The listing builds one solid part. Answer for the finished solid, in the listing's coordinates (mm). Coordinates: 2 decimals unless noted, no trailing zeros. Order: outer loops, then holes, each group sorted by start corner. A loop starts at its lowest first (then second) coordinate and runs counter-clockwise, first axis right, second up. Notation, with made-up numbers: (73.5, 57.25) -> (82.5, 57.25) arc R32 cw to (82.5, 90.25) -> close; hole circle Ø9 at (38, 51). An arc over 180 degrees is marked (long way). One line per question, with ' | ' between items.
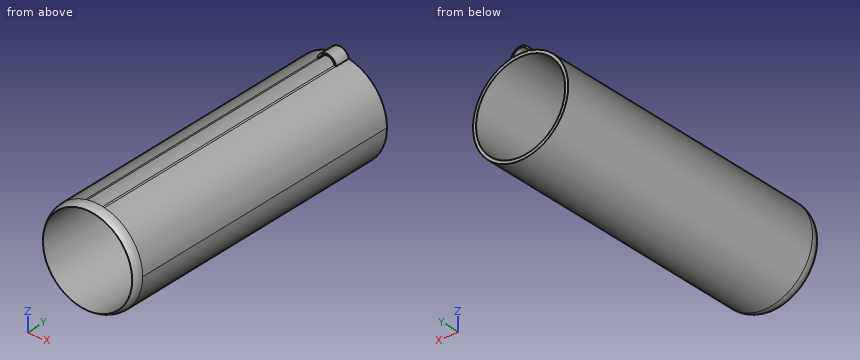
from build123d import *

# Parameters (mm, degrees)
F0_R     = 15
F1_DEPTH = 100
F2_DEPTH = 5


# Not quite as in the source:
# - a fillet or chamfer that OpenCascade refuses, or shapes differently, is made with other operations: its cross-section is extruded or revolved along the edge and cut away or added


with BuildPart() as f1:
    # F0 (on Front) → F1 (new body)
    with BuildSketch(Plane.XZ):
        with BuildLine():
            ThreePointArc((3.1768111268, 15.6814499031), (2.876945892, 15.7392243244), (2.5760326281, 15.7912651773))
            ThreePointArc((2.5760326281, 15.7912651773), (0, 16), (-2.5760326281, 15.7912651773))
            ThreePointArc((-2.5760326281, 15.7912651773), (-2.876945892, 15.7392243244), (-3.1768111268, 15.6814499031))
            ThreePointArc((-3.1768111268, 15.6814499031), (-10.1284505718, -12.3860602701), (16, 0))
            ThreePointArc((16, 0), (12.3860602701, 10.1284505718), (3.1768111268, 15.6814499031))
        make_face()
        Circle(F0_R, mode=Mode.SUBTRACT)
    extrude(amount=F1_DEPTH)

    # F0 (on Front) → F2 (join)
    with BuildSketch(Plane.XZ):
        with BuildLine():
            ThreePointArc((-2.5760326281, 15.7912651773), (0, 17.6948181166), (2.5760326281, 15.7912651773))
            ThreePointArc((2.5760326281, 15.7912651773), (2.876945892, 15.7392243244), (3.1768111268, 15.6814499031))
            ThreePointArc((3.1768111268, 15.6814499031), (0, 18.2490772391), (-3.1768111268, 15.6814499031))
            ThreePointArc((-3.1768111268, 15.6814499031), (-2.876945892, 15.7392243244), (-2.5760326281, 15.7912651773))
        make_face()
        with BuildLine():
            ThreePointArc((3.1768111268, 15.6814499031), (2.876945892, 15.7392243244), (2.5760326281, 15.7912651773))
            ThreePointArc((2.5760326281, 15.7912651773), (0, 16), (-2.5760326281, 15.7912651773))
            ThreePointArc((-2.5760326281, 15.7912651773), (-2.876945892, 15.7392243244), (-3.1768111268, 15.6814499031))
            ThreePointArc((-3.1768111268, 15.6814499031), (-10.1284505718, -12.3860602701), (16, 0))
            ThreePointArc((16, 0), (12.3860602701, 10.1284505718), (3.1768111268, 15.6814499031))
        make_face()
        Circle(F0_R, mode=Mode.SUBTRACT)
    extrude(amount=F2_DEPTH)

    # F3: fillet of radius 5 on 1 edges, made by hand

    # F3_s1 → F3_t2 (revolve, cut)
    with BuildSketch(Plane.XY):
        with BuildLine():
            ThreePointArc((16, -97), (15.7434164903, -98.5811388301), (15, -100))
            Line((15, -100), (16, -100))
            Line((16, -100), (16, -97))
        make_face()
    revolve(axis=Axis((0, -100, 0), (0, 1, 0)), mode=Mode.SUBTRACT)


solid = f1.part
Item 1: Section A-A, the plane x = 0 is taken. Give the vertices of the cut face in (y, z).
Computed values:
outline: (-100, -15) arc R5 ccw to (-97, -16) -> (0, -16) -> (0, -15) -> close; (-100, 15) -> (0, 15) -> (0, 16) -> (-97, 16) arc R5 ccw to start; (-5, 17.69) -> (0, 17.69) -> (0, 18.25) -> (-5, 18.25) -> close
Item 2: Section B-B, the plane y = -48 is taken. Give the vertices of the cut face in (x, z).
Computed values:
outline: circle Ø32 at (0, 0); hole circle Ø30 at (0, 0)
Item 3: Find the intervals of material crossed by L1, parallel to Z at x = 0, y = -52; L2, parallel to X at y = -5, z = 2; L3, parallel to X at y = -30, z = 9.5, in increasing order.
Computed values:
L1: z = -16 to -15, 15 to 16 | L2: x = -15.87 to -14.87, 14.87 to 15.87 | L3: x = -12.87 to -11.61, 11.61 to 12.87
Item 4: Each of these flat-tipped pins is pushed along its axis until it touches: pin 1 Ø2 at (y, z) = (-10, -1) entering from -X; pin 2 Ø1 at (y, z) = (-53, -9.5) entering from +X; pin 3 Ø1.5 at (y, z) = (-78.5, -8.5) entering from +X; pin 4 Ø2 at (x, z) = (1.5, 17.5) entering from -Y. Where does it stop, or does it pass through?
Computed values:
pin 1: stops at x = -16 | pin 2: stops at x = 13.23 | pin 3: stops at x = 14 | pin 4: stops at y = -5
